from build123d import *

# Parameters (mm, degrees)
SKETCH_R     = 2.8
PAD_DEPTH    = 3
SKETCH001_R  = 1.45
PAD001_DEPTH = 30
POCKET_DEPTH = 2
CHAMFER_SIZE = 0.25


with BuildPart() as part:
    # Sketch → Pad (new body)
    with BuildSketch(Plane.XY):
        Circle(SKETCH_R)
    extrude(amount=PAD_DEPTH)

    # Sketch001 (on Face3 of Pad) → Pad001 (join)
    with BuildSketch(Plane.XY.offset(3)):
        Circle(SKETCH001_R)
    extrude(amount=PAD001_DEPTH)

    # Sketch002 (on Face2 of Pad001) → Pocket (cut)
    with BuildSketch(Plane(origin=(0, 0, 0), x_dir=(1, 0, 0), z_dir=(0, 0, -1))):
        Polygon((1.259542, 0.814588), (-0.075682, 1.49809), (-1.335225, 0.683502), (-1.259542, -0.814588), (0.075682, -1.49809), (1.335225, -0.683502), align=None)
    extrude(amount=-POCKET_DEPTH, mode=Mode.SUBTRACT)

    # Chamfer
    chamfer_edges = [part.edges().sort_by_distance(p)[0] for p in [
        (-2.8, 0, 3),
        (-2.8, 0, 0),
        (1.297384, -0.065543, 0),
        (0.705454, 1.090796, 0),
        (-0.59193, 1.156339, 0),
        (-1.297384, 0.065543, 0),
        (-0.705454, -1.090796, 0),
        (0.59193, -1.156339, 0),
        (-1.45, 0, 33),
    ]]
    chamfer(chamfer_edges, length=CHAMFER_SIZE)


solid = part.part
Input: part model. Units: mm. Frame: model coordinates. A direction names the side the tool comes from. Give positions to 0.01 mm unless a question says otherwise; leave off trailing zeros. Order: outer loops, then holes, each group sorted by start corner. A loop starts at its lowest first (then second) coordinate and runs counter-clockwise, first axis right, second up. Notation, with made-up numbers: M -18,68 L 17,68 A30 ccw 17,101 Z; hole C 68,22 d1. An arc over 180 degrees is marked long. Answer as a JSON object with one key per item and string values.
1. Cut plane B-B, the plane z = 19.5. Output: boundary loops of the cut face in (x, y), and give its area (3 significant figures).
Result sheet:
{"outline": "C 0,0 d2.9", "area": "6.61 mm²"}
2. Ray query, line 1 (Z direction, x = -2.2, y = -1.3); line 2 (X direction, y = 0.55, z = 26.5); line 3 (Y direction, x = 0.1, z = 7). Return the intervals inside material, ascending. Write a range as [from, to].
Result sheet:
{"line 1": "[0.01, 2.99]", "line 2": "[-1.34, 1.34]", "line 3": "[-1.45, 1.45]"}
3. Pull-direction query (X, two-part tool) for faces 4 (the flat face through (-0.6, 1.15, 1.11)), 5 (the flat face through (2, 0, 0)), 6 (the cylindrical face through (-1.45, 0.06, 17.67)); classes: +X half, -X half, draft (parallel to the pull), parting line (faces both ways), or undercut.
Result sheet:
{"face 4": "undercut", "face 5": "draft", "face 6": "parting line"}
4. Reachability of faces 1 (the flat face through (0.6, -1.15, 1.11)), 2 (the flat face through (0, -2, 3)), 3 (the flat face through (0, 0, 33)) from +Z, -Z, +X, -X, +Y, -Y: full face, straight path, thin tool, end or side. Return the list, or none.
Result sheet:
{"face 1": "-Z", "face 2": "+Z", "face 3": "+Z, +X, -X, +Y, -Y"}
5. Cut plane A-A, the plane y = 0. Output: boundary loops of the cut face in (x, z).
Result sheet:
{"outline": "M -2.8,0.25 L -2.55,0 L -1.55,0 L -1.3,0.25 L -1.3,2 L 1.3,2 L 1.3,0.25 L 1.55,0 L 2.55,0 L 2.8,0.25 L 2.8,2.75 L 2.55,3 L 1.45,3 L 1.45,32.75 L 1.2,33 L -1.2,33 L -1.45,32.75 L -1.45,3 L -2.55,3 L -2.8,2.75 Z"}
6. First-contact query: P1, Ø2, axis at x = 1, z = 8, coming from the -Y side; P2, Ø0.8, axis at x = -0.5, y = 0, coming from the -Z side; P3, Ø1.5, axis at x = 1.5, y = 2, coming from the +Z side. Flat tips, straight axial feed; report the tip coordinate or a pass-through.
Result sheet:
{"P1": "y = -1.45", "P2": "z = 2", "P3": "z = 3"}
